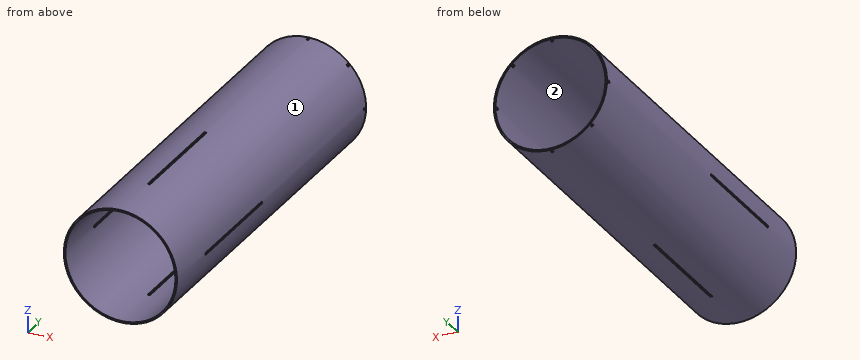
```python
from build123d import *

# Parameters (mm, degrees)
SKETCH1_R           = 78.359
SKETCH1_R_2         = 76.2
BOSS_EXTRUDE1_DEPTH = 508
SKETCH2_W           = 3.175
SKETCH2_H           = 152.4
CUT_EXTRUDE1_DEPTH  = 520.946406625
CIRPATTERN1_COUNT   = 4
SKETCH2_3_R         = 1.750000056
CUT_EXTRUDE2_DEPTH  = 520.946406625
CIRPATTERN2_COUNT   = 8


with BuildPart() as part:
    # Sketch1 → Boss-Extrude1 (new body)
    with BuildSketch(Plane(origin=(0, 0, 0), x_dir=(1, 0, 0), z_dir=(0, 1, 0))):
        with Locations(Location((0, 0, 0), (0, 0, 270))):
            Circle(SKETCH1_R)
        with Locations(Location((0, 0, 0), (0, 0, 270))):
            Circle(SKETCH1_R_2, mode=Mode.SUBTRACT)
    extrude(amount=BOSS_EXTRUDE1_DEPTH)

    # Sketch2 → Cut-Extrude1 (cut, through all)
    with BuildSketch(Plane(origin=(0, 0, 0), x_dir=(0, 0, -1), z_dir=(1, 0, 0))):
        with Locations((0, 152.4)):
            Rectangle(SKETCH2_W, SKETCH2_H)
    cut_extrude1 = extrude(amount=-CUT_EXTRUDE1_DEPTH, mode=Mode.SUBTRACT)

    # CirPattern1: Cut-Extrude1 ×4 about axis
    cirpattern1_axis = Axis((0, 0, 0), (0, 1, 0))
    for i in range(1, CIRPATTERN1_COUNT):
        add(cut_extrude1.rotate(cirpattern1_axis, i * 360 / CIRPATTERN1_COUNT), mode=Mode.SUBTRACT)

    # Sketch2_3 → Cut-Extrude2 (cut, through all)
    with BuildSketch(Plane(origin=(0, 0, 0), x_dir=(0, 0, -1), z_dir=(1, 0, 0))):
        with Locations((0, 503.2375)):
            Circle(SKETCH2_3_R)
    cut_extrude2 = extrude(amount=-CUT_EXTRUDE2_DEPTH, mode=Mode.SUBTRACT)

    # CirPattern2: Cut-Extrude2 ×8 about axis
    cirpattern2_axis = Axis((0, 508, 0), (0, -1, 0))
    for i in range(1, CIRPATTERN2_COUNT):
        add(cut_extrude2.rotate(cirpattern2_axis, i * 360 / CIRPATTERN2_COUNT), mode=Mode.SUBTRACT)


solid = part.part
```
Source: CAD feature listing. Evaluate the final solid. Frame: model axes, mm. Face numbers are marked on the shaded views. Coordinates: 2 decimals unless noted, no trailing zeros. Write each loop counter-clockwise with the first axis right and the second up, starting at its lowest first coordinate (ties: lowest second). Pieces come first, ordered by that corner, then holes. Notation, with made-up numbers: M 86.25,66 L 99.25,66 A11 cw 99.25,70 Z; hole C 85.5,25 d5. An arc over 180 degrees is marked long. Answer as a JSON object with one key per item and string values.
1. Cut plane A-A on z = 44.5. Output: boundary loops of the cut face in (x, y).
Evaluation:
{"outline": "M -64.5,0 L -61.86,0 L -61.86,508 L -64.5,508 Z; M 61.86,0 L 64.5,0 L 64.5,508 L 61.86,508 Z"}
2. Contact query for flat-ended pins moving along their axis: P1, Ø2, axis at x = -55.5, y = 247.5, coming from the +Z side; P2, Ø2, axis at y = 173.5, z = 7.5, coming from the -X side; P3, Ø3, axis at y = 503.24, z = 0, coming from the +X side; P4, Ø1, axis at x = 36, y = 295, coming from the -Z side. Output: stop coordinate, or through.
Evaluation:
{"P1": "z = 56.3", "P2": "x = -78.09", "P3": "through", "P4": "z = -69.86"}
3. Draft query along X for the marked faces 1 and 2. Return one class per face: released by +X, released by -X, zero draft, split by the parting line, or undercut.
Evaluation:
{"face 1": "split by the parting line", "face 2": "undercut"}
4. Ray query, L1, parallel to Y at x = -77.05, z = 0; L2, parallel to X at y = 239, z = 0; L3, parallel to Z at x = -42, y = 177. Return the intervals inside material, ascending.
Evaluation:
{"L1": "0 to 76.2, 228.6 to 501.49, 504.99 to 508", "L2": "-78.36 to -76.2, 76.2 to 78.36", "L3": "-66.15 to -63.58, 63.58 to 66.15"}
5. Cut plane B-B on x = -61.5. Output: boundary loops of the cut face in (y, z).
Evaluation:
{"outline": "M 0,-48.56 L 508,-48.56 L 508,-44.99 L 0,-44.99 Z; M 0,44.99 L 508,44.99 L 508,48.56 L 0,48.56 Z"}
